Source: three-view drawing plus pictorial views. Frame: mm from the lowest corner of the part. Give positions to 0.01 mm unless a question says otherwise; leave off trailing zeros. Order: outer loops, then holes, each group sorted by start corner. A loop starts at its lowest first (then second) coordinate and runs counter-clockwise, first axis right, second up. Notation, with made-up numbers: (71, -20.5) -> (110, -20.5) arc R26 ccw to (110, -3.5) -> close; hole circle Ø6 at (54.5, 67.25). An arc over 180 degrees is marked (long way). One line per question, with ' | ' between items.
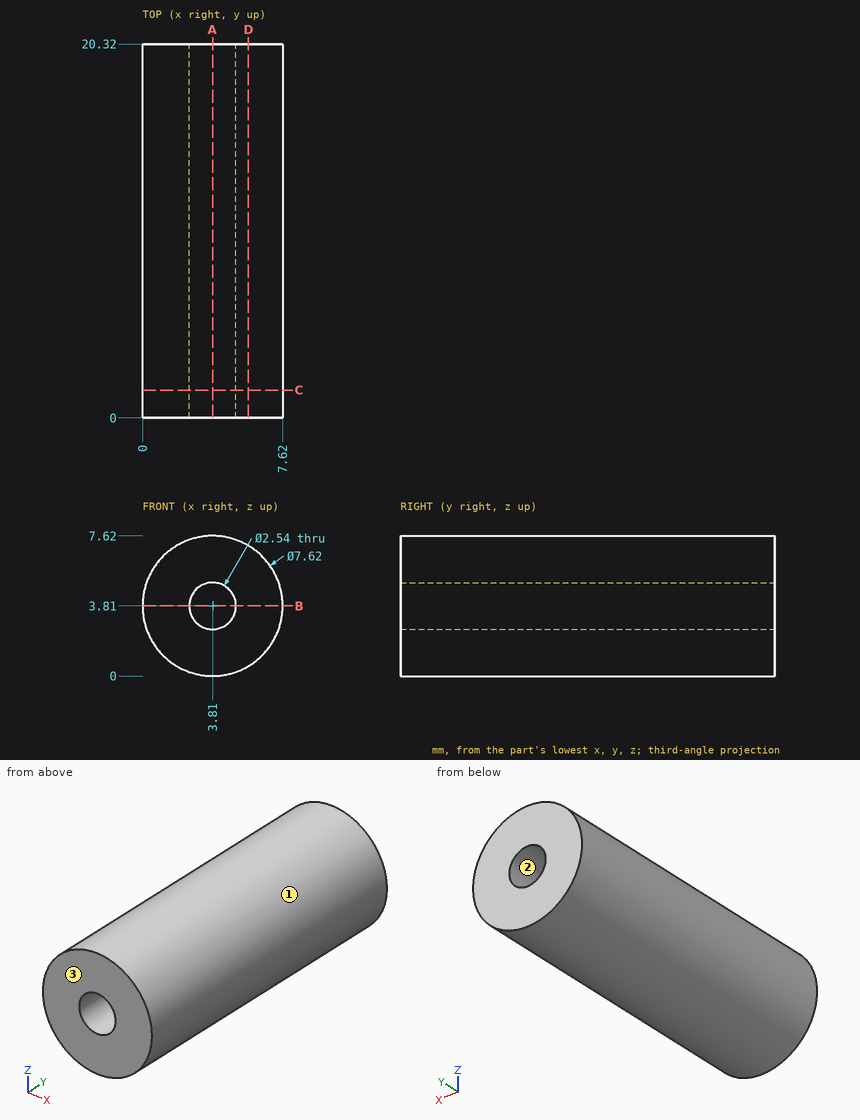
1) Pull-direction query (X, two-part tool) for the marked faces 1, 2 and 3; classes: +X half, -X half, draft (parallel to the pull), parting line (faces both ways), or undercut.
Check result:
face 1: parting line | face 2: undercut | face 3: draft
2) Contact query for flat-ended pins moving along their axis: pin 1 Ø3 at (y, z) = (13, 3) entering from -X; pin 2 Ø2 at (x, z) = (3.81, 3.81) entering from +Y; pin 3 Ø1 at (x, y) = (1, 17) entering from +Z. Output: stop coordinate, or through.
Check result:
pin 1: stops at x = 0 | pin 2: passes through | pin 3: stops at z = 6.84
3) Section A-A on x = 3.81. Return loops of the section in (y, z).
Check result:
outline: (0, 0) -> (20.32, 0) -> (20.32, 2.54) -> (0, 2.54) -> close; (0, 5.08) -> (20.32, 5.08) -> (20.32, 7.62) -> (0, 7.62) -> close
4) Section C-C on y = 1.5. Return loops of the section in (x, z), plus the area to 3 significant figures.
Check result:
outline: circle Ø7.62 at (3.81, 3.81); hole circle Ø2.54 at (3.81, 3.81) | area: 40.5 mm^2
5) Section B-B on z = 3.81. Return loops of the section in (x, y), plus the area to 3 significant figures.
Check result:
outline: (0, 0) -> (2.54, 0) -> (2.54, 20.32) -> (0, 20.32) -> close; (5.08, 0) -> (7.62, 0) -> (7.62, 20.32) -> (5.08, 20.32) -> close | area: 103 mm^2
6) Material intervals for probe 1 along Z at (x, y) = (3.81, 7.75); probe 2 along X at (y, z) = (10.75, 3.5); probe 3 along Z at (x, y) = (4.5, 18.5), sorted ascending. Write a range as from..to.
Check result:
probe 1: z = 0..2.54, 5.08..7.62 | probe 2: x = 0.01..2.58, 5.04..7.61 | probe 3: z = 0.06..2.74, 4.88..7.56
7) Section D-D on x = 5.75. Return loops of the section in (y, z), plus the area to 3 significant figures.
Check result:
outline: (0, 0.53) -> (20.32, 0.53) -> (20.32, 7.09) -> (0, 7.09) -> close | area: 133 mm^2
